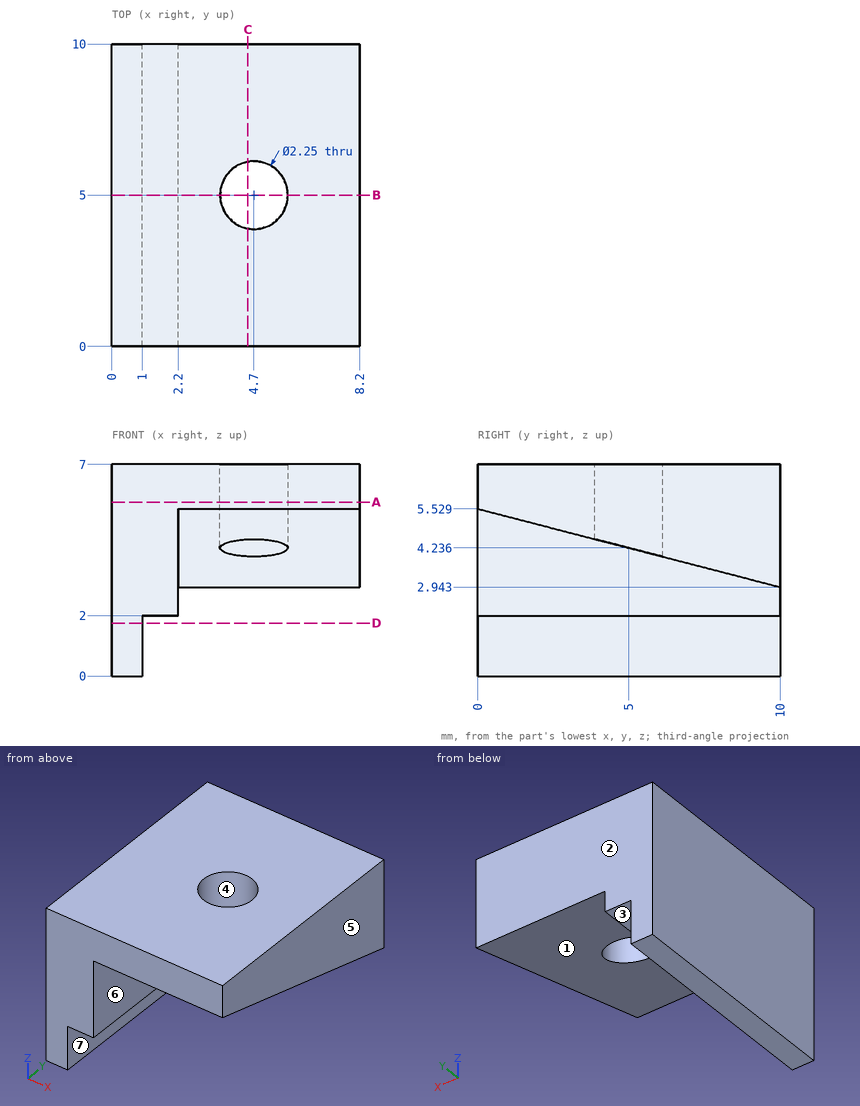
Here's the drawing with two shaded views (mm, measured from the low corner). I have some questions. A direction names the side the tool comes from. Coordinates: 2 decimals unless noted, no trailing zeros. Loops run counter-clockwise (first coordinate to the right, second up) from the corner with the lowest first, then second, coordinate; pieces in that order, holes last. Notation, with made-up numbers: (27, 11.5) -> (32, 11.5) arc R30 cw to (32, 41.5) -> close; hole circle Ø5 at (19.5, 29). An arc over 180 degrees is marked (long way). Answer as a JSON object with one key per item and string values.
1) For P1, Ø4, axis at x = 3.5, y = 4.5, coming from the -Z side; P2, Ø2, axis at y = 8, z = 2, coming from the +X side; P3, Ø2, axis at x = 4.7, y = 5, coming from the +Z side; P4, Ø2, axis at y = 3.5, z = 0.5, coming from the +X side, each with a flat end and sliding along its axis, tell me the tip position at first contact or that it passes through.
Results:
{"P1": "stops at z = 2", "P2": "stops at x = 2.2", "P3": "passes through", "P4": "stops at x = 1"}
2) Imagine slicing it at D-D (z = 1.75). Please give me the cut outline in (x, y).
Results:
{"outline": "(0, 0) -> (1, 0) -> (1, 10) -> (0, 10) -> close"}
3) For the marked faces 5, 6 and 7, which set-ups out of +Z, -Z, +X, -X, +Y, -Y let a thin tool reach every point of the face, with its end or its side?
Results:
{"face 5": "+Z, -Z, +X, +Y, -Y", "face 6": "-Z, +X, -Y", "face 7": "-Z, +X, +Y, -Y"}
4) Imagine slicing it at A-A (z = 5.75). Please give me the cut outline in (x, y) (3 decimals).
Results:
{"outline": "(0, 0) -> (8.2, 0) -> (8.2, 10) -> (0, 10) -> close; hole circle Ø2.25 at (4.7, 5)"}
5) Thinking about a two-plate mould opening in Y: for the marked faces 1, 2, 3 and 4, which applies, pulls with the +Y half, pulls with the -Y half, needs draft (parallel to the pull), parting line crosses it, or undercut?
Results:
{"face 1": "pulls with the -Y half", "face 2": "pulls with the +Y half", "face 3": "needs draft", "face 4": "undercut"}
6) Imagine slicing it at C-C (x = 4.5). Please give me the cut outline in (y, z).
Results:
{"outline": "(0, 5.53) -> (3.89, 4.52) -> (3.89, 7) -> (0, 7) -> close; (6.11, 3.95) -> (10, 2.94) -> (10, 7) -> (6.11, 7) -> close"}
7) If I drill on line 1 (X direction, y = 5, z = 5.85) (3 decimals); line 2 (Y direction, x = 4.7, z = 6.1) (3 decimals); line 3 (Z direction, x = 2, y = 4.5), over which ranges is the centre line in solid material (lowest first)?
Results:
{"line 1": "x = 0 to 3.575, 5.825 to 8.2", "line 2": "y = 0 to 3.875, 6.125 to 10", "line 3": "z = 2 to 7"}
8) Imagine slicing it at B-B (y = 5). Please give me the cut outline in (x, z) (3 decimals).
Results:
{"outline": "(0, 0) -> (1, 0) -> (1, 2) -> (2.2, 2) -> (2.2, 4.236) -> (3.575, 4.236) -> (3.575, 7) -> (0, 7) -> close; (5.825, 4.236) -> (8.2, 4.236) -> (8.2, 7) -> (5.825, 7) -> close"}
